Geometry check sheet. Reference: the model listing, model coordinates, mm. A direction names the side the tool comes from. Coordinates: 2 decimals unless noted, no trailing zeros. Write each loop counter-clockwise with the first axis right and the second up, starting at its lowest first coordinate (ties: lowest second). Pieces come first, ordered by that corner, then holes. Notation, with made-up numbers: (-33, 30) -> (-4, 30) arc R11 cw to (-4, 43) -> close; hole circle Ø2 at (12, -2.5). An arc over 180 degrees is marked (long way). One line per question, with ' | ' between items.
```python
from build123d import *

# Parameters (mm, degrees)
F1_DEPTH = 177.8
F2_T     = -12.7
F3_R     = 6.7589749521
F4_DEPTH = 0.0762


with BuildPart() as f1:
    # F0 (on Top) → F1 (new body)
    with BuildSketch(Plane.XY):
        Polygon((42.9860351945, -4.42373426), (17.4906366902, 39.5151398165), (-32.1762272351, 28.8454337368), (-37.3766387512, -21.687681347), (9.0761941016, -42.2491579463), align=None)
    extrude(amount=F1_DEPTH)

    # F2
    f2_openings = [f1.faces().sort_by_distance(p)[0] for p in [
        (0, 0, 177.8),
    ]]
    offset(amount=F2_T, openings=f2_openings)

    # F3 (on face) → F4 (cut)
    with BuildSketch(Plane(origin=(-7.3427952725, 34.1802867766, 0), x_dir=(-0.9776941718, -0.2100335842, 0), z_dir=(-0.2100335842, 0.9776941718, 0))):
        with Locations((0, 81.7129537463)):
            Circle(F3_R)
    extrude(amount=-F4_DEPTH, mode=Mode.SUBTRACT)


solid = f1.part
```
(1) Material ranges on line 1 (X direction, y = 17.5, z = 103.5); line 2 (Y direction, x = -7, z = 162.5); line 3 (Z direction, x = 12.5, y = 22.5), recorded low to high.
Answers below:
line 1: x = -33.34 to -20.58, 15.58 to 30.26 | line 2: y = -35.13 to -21.24, 21.26 to 34.25 | line 3: z = 0 to 12.7
(2) Depth check by flat-ended pin: P1, Ø1, axis at y = -7.5, z = 80, coming from the -X side; P2, Ø10, axis at y = 3, z = 85, coming from the +X side; P3, Ø3, axis at x = 2, y = -31, coming from the -Z side; P4, Ø1.5, axis at y = -5.5, z = 23.5, coming from the +X side. Enter the tip coordinate at first touch or a pass-through.
Answers below:
P1: stops at x = -35.97 | P2: stops at x = 41.58 | P3: stops at z = 0 | P4: stops at x = 42.69
(3) Cross-section at D-D (y = -33.5). Record the cut outline in (x, z).
Answers below:
outline: (-10.69, 0) -> (16.92, 0) -> (16.92, 177.8) -> (-10.69, 177.8) -> close
(4) Cross-section at A-A (z = 134). Record the cut outline in (x, y), plus the area to 3 significant figures.
Answers below:
outline: (-37.38, -21.69) -> (9.08, -42.25) -> (42.99, -4.42) -> (17.49, 39.52) -> (-32.18, 28.85) -> close; hole (-23.8, -13.81) -> (5.78, -26.9) -> (27.37, -2.82) -> (11.14, 25.16) -> (-20.49, 18.37) -> close | area: 2,640 mm²
(5) Cross-section at B-B (y = 11). Record the cut outline in (x, z).
Answers below:
outline: (-34.01, 0) -> (34.04, 0) -> (34.04, 177.8) -> (19.35, 177.8) -> (19.35, 12.7) -> (-21.25, 12.7) -> (-21.25, 177.8) -> (-34.01, 177.8) -> close
(6) Cross-section at C-C (x = 13). Record the cut outline in (y, z), plus the area to 3 significant figures.
Answers below:
outline: (-37.87, 0) -> (38.55, 0) -> (38.55, 177.8) -> (21.95, 177.8) -> (21.95, 12.7) -> (-18.85, 12.7) -> (-18.85, 177.8) -> (-37.87, 177.8) -> close | area: 6,850 mm²
(7) Draft check along Y on faces 3 (the face through (-7.234, 34.126, 81.808)), 4 (the face through (2, -1, 0)), 5 (the face through (16.42, -15.03, 94.09)). Enter one of: pulls with the +Y half, pulls with the -Y half, needs draft (parallel to the pull), parting line crosses it, or undercut.
Answers below:
face 3: pulls with the +Y half | face 4: needs draft | face 5: undercut
(8) Tool access check on faces 1 (the face through (-16, -19, 177.8)), 2 (the face through (19.367, 10.976, 94.094)). Record the directions out of +Z, -Z, +X, -X, +Y, -Y that give a thin tool (end or side, any length) a straight path to the whole face; none if there is none.
Answers below:
face 1: +Z, +X, -X, +Y, -Y | face 2: +Z
